from build123d import *

# Parameters (mm, degrees)
SKETCH1_R           = 4
SKETCH1_R_2         = 0.5
SKETCH1_R_3         = 1.5
BOSS_EXTRUDE1_DEPTH = 4


with BuildPart() as part:
    # Sketch1 → Boss-Extrude1 (new body)
    with BuildSketch(Plane.XY):
        with BuildLine():
            Line((12, 24), (133, 24))
            ThreePointArc((133, 24), (145, 12), (133, 0))
            Line((133, 0), (12, 0))
            ThreePointArc((12, 0), (0, 12), (12, 24))
        make_face()
        with Locations((133, 12)):
            Circle(SKETCH1_R, mode=Mode.SUBTRACT)
        with Locations((133, 19.4)):
            Circle(SKETCH1_R_2, mode=Mode.SUBTRACT)
        with Locations((133.121025162, 4.600989734)):
            Circle(SKETCH1_R_2, mode=Mode.SUBTRACT)
        with Locations((140.4, 12)):
            Circle(SKETCH1_R_2, mode=Mode.SUBTRACT)
        with Locations((125.6, 12)):
            Circle(SKETCH1_R_2, mode=Mode.SUBTRACT)
        with Locations((60, 5)):
            Circle(SKETCH1_R_3, mode=Mode.SUBTRACT)
        with Locations((60, 19)):
            Circle(SKETCH1_R_3, mode=Mode.SUBTRACT)
        with Locations((85, 5)):
            Circle(SKETCH1_R_3, mode=Mode.SUBTRACT)
        with Locations((85, 19)):
            Circle(SKETCH1_R_3, mode=Mode.SUBTRACT)
        with Locations((12, 12)):
            Circle(SKETCH1_R, mode=Mode.SUBTRACT)
        with Locations((12, 4.6)):
            Circle(SKETCH1_R_2, mode=Mode.SUBTRACT)
        with Locations((11.878974838, 19.399010266)):
            Circle(SKETCH1_R_2, mode=Mode.SUBTRACT)
        with Locations((4.6, 12)):
            Circle(SKETCH1_R_2, mode=Mode.SUBTRACT)
        with Locations((19.4, 12)):
            Circle(SKETCH1_R_2, mode=Mode.SUBTRACT)
    extrude(amount=BOSS_EXTRUDE1_DEPTH)


solid = part.part
Build history of the part. All positions in model axes, mm. Round coordinates to 2 decimals unless told otherwise and drop trailing zeros. Loops run counter-clockwise (first coordinate to the right, second up) from the corner with the lowest first, then second, coordinate; pieces in that order, holes last. Notation, with made-up numbers: (-10.75, 27.5) -> (45.25, 27.5) arc R21 ccw to (45.25, 65.5) -> close; hole circle Ø6 at (50.25, -15). An arc over 180 degrees is marked (long way). Answer in a Markdown table with one row per item.
Item 1: Mould opens along Y. For faces 1 (the cylindrical face through (86.43, 19.45, 1.97)), 2 (the flat face through (74, 12, 4)), 3 (the cylindrical face through (0, 12, 2)) say: +Y half, -Y half, draft (parallel to the pull), parting line (faces both ways), or undercut.
Answers below:
| item | result |
|---|---|
| face 1 | undercut |
| face 2 | draft |
| face 3 | parting line |
Item 2: Saw through at B-B (z = 2.55). State how many separate pieces and enclosed holes the cut face has, and give its area (3 significant figures).
Answers below:
| item | result |
|---|---|
| separate pieces | 1 |
| enclosed holes | 14 |
| area | 3,220 mm² |
Item 3: Saw through at A-A (y = 10). Write the cut outline in (x, z).
Answers below:
| item | result |
|---|---|
| outline | (0.17, 0) -> (8.54, 0) -> (8.54, 4) -> (0.17, 4) -> close; (15.46, 0) -> (129.54, 0) -> (129.54, 4) -> (15.46, 4) -> close; (136.46, 0) -> (144.83, 0) -> (144.83, 4) -> (136.46, 4) -> close |
Item 4: Drill centre lines: L1, parallel to Y at x = 60, z = 2.35; L2, parallel to Y at x = 19.4, z = 2.85; L3, parallel to Y at x = 12, z = 1.65. Where is each one in solid material? Low to high. Write a range as [from, to].
Answers below:
| item | result |
|---|---|
| L1 | y = [0, 3.5], [6.5, 17.5], [20.5, 24] |
| L2 | y = [0, 11.5], [12.5, 24] |
| L3 | y = [0, 4.1], [5.1, 8], [16, 18.91], [19.88, 24] |
Item 5: Pin check, flat tip, straight feed: pin 1 (1.5 mm diameter, centred on y = 14, z = 1.5, fed in from +X). Stop position of the tip, or through.
Answers below:
| item | result |
|---|---|
| pin 1 | stops at x = 144.93 |
Item 6: Saw through at C-C (y = 22). Write the cut outline in (x, z), and give its area (3 significant figures).
Answers below:
| item | result |
|---|---|
| outline | (5.37, 0) -> (139.63, 0) -> (139.63, 4) -> (5.37, 4) -> close |
| area | 537 mm² |
